Could you check a few things on this model? Use its own coordinates, in mm. Face numbers are marked on the shaded views. Coordinates: 2 decimals unless noted, no trailing zeros. Order: outer loops, then holes, each group sorted by start corner. A loop starts at its lowest first (then second) coordinate and runs counter-clockwise, first axis right, second up. Notation, with made-up numbers: M 48,79.25 L 87,79.25 A19 ccw 87,98.25 Z; hole C 39,-9.75 d8. An arc over 180 degrees is marked long. Put each result on its own line as item: value. Start each with the question number.
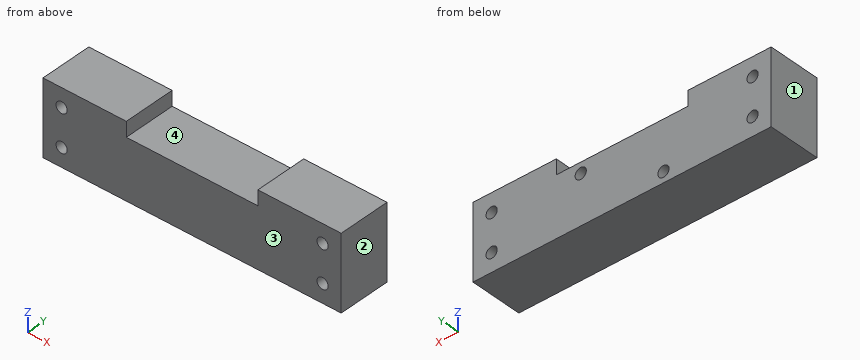
```python
from build123d import *

# Parameters (mm, degrees)
SKETCH1_W           = 80
SKETCH1_H           = 14
BOSS_EXTRUDE1_DEPTH = 20
SKETCH2_W           = 35.292
SKETCH2_H           = 14
CUT_EXTRUDE1_DEPTH  = 4
SKETCH3_R           = 1.5
CUT_EXTRUDE2_DEPTH  = 14
SKETCH4_R           = 1.5
CUT_EXTRUDE3_DEPTH  = 8


with BuildPart() as part:
    # Sketch1 → Boss-Extrude1 (new body)
    with BuildSketch(Plane.XY):
        with Locations((40, 7)):
            Rectangle(SKETCH1_W, SKETCH1_H)
    extrude(amount=BOSS_EXTRUDE1_DEPTH)

    # Sketch2 → Cut-Extrude1 (cut)
    with BuildSketch(Plane.XY.offset(20)):
        with Locations((40, 7)):
            Rectangle(SKETCH2_W, SKETCH2_H)
    extrude(amount=-CUT_EXTRUDE1_DEPTH, mode=Mode.SUBTRACT)

    # Sketch3 → Cut-Extrude2 (cut)
    with BuildSketch(Plane(origin=(0, 14, 0), x_dir=(1, 0, 0), z_dir=(0, 1, 0))):
        with Locations((5, -5)):
            Circle(SKETCH3_R)
        with Locations((5, -15)):
            Circle(SKETCH3_R)
        with Locations((75, -15)):
            Circle(SKETCH3_R)
        with Locations((75, -5)):
            Circle(SKETCH3_R)
    extrude(amount=-CUT_EXTRUDE2_DEPTH, mode=Mode.SUBTRACT)

    # Sketch4 → Cut-Extrude3 (cut)
    with BuildSketch(Plane(origin=(0, 14, 0), x_dir=(1, 0, 0), z_dir=(0, 1, 0))):
        with Locations((28.9, -2.87)):
            Circle(SKETCH4_R)
        with Locations((51.1, -13.17)):
            Circle(SKETCH4_R)
    extrude(amount=-CUT_EXTRUDE3_DEPTH, mode=Mode.SUBTRACT)


solid = part.part
```
Item 1: I need wall thicknesses on probe 1 along X at (y, z) = (11.25, 5); probe 2 along Z at (x, y) = (75, 6); probe 3 along Z at (x, y) = (28.9, 8.5). Which ranges of each line are inside material? Lowest first, please.
Item 2: For pin 1 Ø4 at (x, y) = (36, 6.5) entering from +Z, with a flat end and sliding along its axis, tell me the tip position at first contact or that it passes through.
Item 3: If we section it at C-C on x = 28.9: Write out the boundary of the cut face in (y, z).
Item 4: If we section it at A-A on x = 5: Write out the boundary of the cut face in (y, z), then the cut area to 3 significant figures.
Item 5: If we section it at B-B on y = 12: Write out the boundary of the cut face in (x, z), then the cut area to 3 significant figures.
Item 6: If we mould it in two halves opening along X, with no side actions, what happens to the marked faces 1, 2, 3 and 4? For each: released by +X, released by -X, zero draft, split by the parting line, or undercut.
Geometry check:
1. probe 1: x = 0 to 3.5, 6.5 to 73.5, 76.5 to 80
1. probe 2: z = 0 to 3.5, 6.5 to 13.5, 16.5 to 20
1. probe 3: z = 0 to 1.37, 4.37 to 16
2. pin 1: stops at z = 16
3. outline: M 0,0 L 14,0 L 14,1.37 L 6,1.37 L 6,4.37 L 14,4.37 L 14,16 L 0,16 Z
4. outline: M 0,0 L 14,0 L 14,3.5 L 0,3.5 Z; M 0,6.5 L 14,6.5 L 14,13.5 L 0,13.5 Z; M 0,16.5 L 14,16.5 L 14,20 L 0,20 Z
4. area: 196 mm²
5. outline: M 0,0 L 80,0 L 80,20 L 57.65,20 L 57.65,16 L 22.35,16 L 22.35,20 L 0,20 Z; hole C 5,5 d3; hole C 5,15 d3; hole C 28.9,2.87 d3; hole C 51.1,13.17 d3; hole C 75,5 d3; hole C 75,15 d3
5. area: 1,420 mm²
6. face 1: released by -X
6. face 2: released by +X
6. face 3: zero draft
6. face 4: undercut
